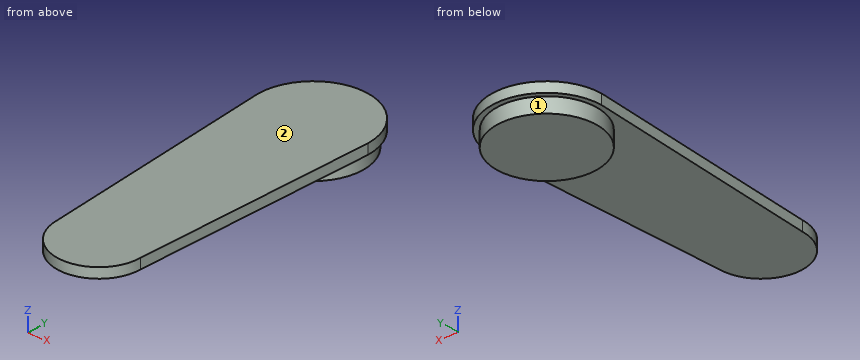
```python
from build123d import *

# Parameters (mm, degrees)
BOSS_EXTRUDE1_DEPTH      = 10
BOSS_EXTRUDE1_DEPTH_BACK = 0.0001
SKETCH2_R                = 50
BOSS_EXTRUDE2_DEPTH      = 15


with BuildPart() as part:
    # Sketch1 → Boss-Extrude1 (new, two sides: drawn at the far end of the back side and taken through both)
    with BuildSketch(Plane.XY.offset(-BOSS_EXTRUDE1_DEPTH_BACK)):
        with BuildLine():
            ThreePointArc((55, 0), (0, 55), (-55, 0))
            Line((-55, 0), (-40.768073077, -239.675921097))
            ThreePointArc((-40.768073077, -239.675921097), (0.881926923, -281.325921097), (42.531926923, -239.675921097))
            Line((42.531926923, -239.675921097), (55, 0))
        make_face()
    extrude(amount=BOSS_EXTRUDE1_DEPTH + BOSS_EXTRUDE1_DEPTH_BACK)

    # Sketch2 → Boss-Extrude2 (add)
    with BuildSketch(Plane(origin=(0, 0, -0.0001), x_dir=(-1, 0, 0), z_dir=(0, 0, -1))):
        with Locations(Location((0, 0, 0), (0, 0, 180))):
            Circle(SKETCH2_R)
    extrude(amount=BOSS_EXTRUDE2_DEPTH)


solid = part.part
```
Here's how the part is built. I have some questions about the finished solid (model axes, mm). Face numbers are marked on the shaded views. A direction names the side the tool comes from. Coordinates: 2 decimals unless noted, no trailing zeros. Loops run counter-clockwise (first coordinate to the right, second up) from the corner with the lowest first, then second, coordinate; pieces in that order, holes last. Notation, with made-up numbers: (63, -9) - (75, -9) arc R8 ccw to (75, 2) - close; hole circle Ø10 at (-18, 37). An arc over 180 degrees is marked (long way). Answer as CSV lines item,"result".
Q1. For pin 1 (3 mm diameter, centred on x = 1.5, z = 5, fed in from -Y); pin 2 (10 mm diameter, centred on y = -91.5, z = 3.5, fed in from -X); pin 3 (5 mm diameter, centred on y = -23.5, z = -9, fed in from -X); pin 4 (10 mm diameter, centred on y = -229, z = -6.5, fed in from +X), each with a flat end and sliding along its axis, tell me the tip position at first contact or that it passes through.
Response:
pin 1,"y = -281.33"
pin 2,"x = -49.86"
pin 3,"x = -45.38"
pin 4,"through"
Q2. If we section it at B-B, the plane z = -5.25: Write out the boundary of the cut face in (x, y).
Response:
outline,"circle Ø100 at (0, 0)"
Q3. If I drill on L1, parallel to Z at x = -15, y = -257; L2, parallel to Y at x = -9, z = -8.75; L3, parallel to X at y = -4, z = -7.5, over which ranges is the centre line in solid material (lowest first)? Write a range as [from, to].
Response:
L1,"[0, 10]"
L2,"[-49.18, 49.18]"
L3,"[-49.84, 49.84]"
Q4. For the marked faces 1 and 2, which set-ups out of +Z, -Z, +X, -X, +Y, -Y let a thin tool reach every point of the face, with its end or its side?
Response:
face 1,"-Z"
face 2,"+Z, +X, -X, +Y, -Y"
Q5. If we section it at D-D, the plane x = -16.5: Write out the boundary of the cut face in (y, z), and give its area (3 significant figures).
Response:
outline,"(-277.53, 0) - (-47.2, 0) - (-47.2, -15) - (47.2, -15) - (47.2, 0) - (52.47, 0) - (52.47, 10) - (-277.53, 10) - close"
area,"4,720 mm2"
Q6. If we section it at A-A, the plane x = 0: Write out the boundary of the cut face in (y, z), and give its area (3 significant figures).
Response:
outline,"(-281.32, 0) - (-50, 0) - (-50, -15) - (50, -15) - (50, 0) - (55, 0) - (55, 10) - (-281.32, 10) - close"
area,"4,860 mm2"
Q7. If we section it at C-C, the plane y = -91: Write out the boundary of the cut face in (x, z).
Response:
outline,"(-49.6, 0) - (50.27, 0) - (50.27, 10) - (-49.6, 10) - close"
